Source: CAD feature listing. Evaluate the final solid. Frame: model axes, mm. A direction names the side the tool comes from. Coordinates: 2 decimals unless noted, no trailing zeros. Order: outer loops, then holes, each group sorted by start corner. A loop starts at its lowest first (then second) coordinate and runs counter-clockwise, first axis right, second up. Notation, with made-up numbers: (12, -26.5) -> (57, -26.5) arc R16 cw to (57, -13.5) -> close; hole circle Ø4 at (89.25, 64.25). An arc over 180 degrees is marked (long way). Put each result on its own line as item: value.
Autodesk Inventor part; units mm, degrees
ref_plane "РабПлоскость2" through (-7.5, 5, 1.5) normal (0, 0, 1) x (1, 0, 0)
ref_plane "YZ Plane" through (0, 0, 0) normal (1, 0, 0) x (0, 1, 0)
ref_plane "XZ Plane" through (0, 0, 0) normal (0, 1, 0) x (-1, 0, 0)
sketch "Эскиз1" plane through (0, 0, 0) normal (0, 1, 0) x (-1, 0, 0)
  line L0 (-10, 1.75) -> (10, 1.75)
  line L1 (10, 1.75) -> (10, -1.75)
  line L2 (10, -1.75) -> (-10, -1.75)
  line L3 (-10, -1.75) -> (-10, 1.75)
  line L4 (-10, 1.75) -> (10, -1.75) construction
  line L5 (10, 1.75) -> (-10, -1.75) construction
  line L6 (2.5, -1.75) -> (-2.5, -1.75)
  line L7 (-2.5, -1.75) -> (-2.5, -3.75)
  line L8 (-2.5, -3.75) -> (2.5, -3.75)
  line L9 (2.5, -3.75) -> (2.5, -1.75)
  line L10 (0, 1.75) -> (0, -1.75)
  point P0 (0, 0)
  dimension "d0" = 20
  dimension "d1" = 3.5
  dimension "d2" = 5
  dimension "d3" = 2
revolve "Вращение1" add sketch "Эскиз1" angle 360 about axis through (0, 0, 1.75) along (0, 0, -1) contours L0 L1 L2 L10
ref_plane "РабПлоскость2" through (-7.5, 5, 1.5) normal (0, 0, 1) x (1, 0, 0)
sketch "Эскиз3" plane through (-7.5, 5, 1.5) normal (0, 0, 1) x (1, 0, 0)
  circle A0 centre (7.5, -5) radius 2.725 construction
  line L0 (7.5, -5) -> (8.8625, -2.6401) construction
  line L1 (7.5, -5) -> (6.1375, -2.6401) construction
  line L2 (7.5, -5) -> (4.775, -5) construction
  line L3 (7.5, -5) -> (6.1375, -7.3599) construction
  line L4 (7.5, -5) -> (8.8625, -7.3599) construction
  line L5 (7.5, -5) -> (10.225, -5) construction
  line L6 (6.1375, -2.6401) -> (8.8625, -2.6401)
  line L7 (8.8625, -2.6401) -> (10.225, -5)
  line L8 (10.225, -5) -> (8.8625, -7.3599)
  line L9 (6.1375, -7.3599) -> (8.8625, -7.3599)
  line L10 (4.775, -5) -> (6.1375, -7.3599)
  line L11 (4.775, -5) -> (6.1375, -2.6401)
  dimension "d12" = 5.45
  dimension "d15" = 360
extrude "Выдавливание4" cut sketch "Эскиз3" along normal blind 2.5 and the other way blind 2.5
sketch "Эскиз4" plane through (0, 0, -1.75) normal (0, 0, -1) x (-1, 0, 0)
  circle A0 centre (0, 0) radius 1.3
  circle A1 centre (0, 0) radius 4.5
  point P0 (0, 0)
  dimension "d20" = 2.6
  dimension "d21" = 9
extrude "Выдавливание5" add sketch "Эскиз4" along normal blind 2
extrude "Выдавливание6" cut sketch "Эскиз4" against normal mid plane 12 contours A0
fillet "Сопряжение1" radius 0.5 1 edges at (10, 0, 1.75)
properties part number "kikcer_head_002"
1. Cut plane C-C on z = -1.3. Output: boundary loops of the cut face in (x, y).
Numbers:
outline: circle Ø20 at (0, 0); hole circle Ø2.6 at (0, 0)
2. Cut plane B-B on z = 0.1. Output: boundary loops of the cut face in (x, y) (1 decimal).
Numbers:
outline: circle Ø20 at (0, 0); hole (-2.7, 0) -> (-1.4, -2.4) -> (1.4, -2.4) -> (2.7, 0) -> (1.4, 2.4) -> (-1.4, 2.4) -> close
3. First-contact query: pin 1 (1.6 mm diameter, centred on x = 0, y = 0, fed in from +Z); pin 2 (1.5 mm diameter, centred on x = 6.5, z = 0, fed in from +Y); pin 3 (1.5 mm diameter, centred on x = 3.5, y = -5, fed in from -Z); pin 4 (5 mm diameter, centred on x = -0.5, y = 1, fed in from +Z). Flat tips, straight axial feed; report the tip coordinate or a pass-through.
Numbers:
pin 1: passes through
pin 2: stops at y = 8.18
pin 3: stops at z = -1.75
pin 4: stops at z = 1.75
4. Set-up query: faces 1 (the flat face through (2.053, -1.163, 0.356)), 2 (the flat face through (-4.3, -2.1, -1.75)), 3 (the cylindrical face through (2.17, -9.76, -0.27)). Return all of +Z, -Z, +X, -X, +Y, -Y with unobstructed straight access to the full face (end or side cutting, diameter ignored); none if empty.
Numbers:
face 1: +Z
face 2: -Z
face 3: +Z, -Z
5. Pull-direction query (Y, two-part tool) for faces 4 (the flat face through (0, -2.36, 0)), 5 (the flat face through (1.1, 1.1, -3.75)), 6 (the cylindrical face through (0.59, -4.46, -2.74)); classes: pulls with the +Y half, pulls with the -Y half, needs draft (parallel to the pull), parting line crosses it, or undercut.
Numbers:
face 4: undercut
face 5: needs draft
face 6: parting line crosses it
6. Cut plane A-A on x = 0. Output: boundary loops of the cut face in (y, z).
Numbers:
outline: (-10, -1.75) -> (-4.5, -1.75) -> (-4.5, -3.75) -> (-1.3, -3.75) -> (-1.3, -1) -> (-2.36, -1) -> (-2.36, 1.75) -> (-9.5, 1.75) arc R0.5 ccw to (-10, 1.25) -> close; (1.3, -3.75) -> (4.5, -3.75) -> (4.5, -1.75) -> (10, -1.75) -> (10, 1.25) arc R0.5 ccw to (9.5, 1.75) -> (2.36, 1.75) -> (2.36, -1) -> (1.3, -1) -> close
7. Ray query, line 1 along Y through (x, z) = (0, -2.7); line 2 along Z through (x, y) = (-4.5, 3); line 3 along X through (y, z) = (-2.25, 0.15). Return the intervals inside material, ascending.
Numbers:
line 1: y = -4.5 to -1.3, 1.3 to 4.5
line 2: z = -1.75 to 1.75
line 3: x = -9.74 to -1.43, 1.43 to 9.74
